Input: dimensioned drawing with shaded views. Units: mm. Origin: part minimum x, y, z. Round coordinates to 2 decimals unless told otherwise and drop trailing zeros. Loops run counter-clockwise (first coordinate to the right, second up) from the corner with the lowest first, then second, coordinate; pieces in that order, holes last.
Item 1: First-contact query: P1, Ø1.4, axis at y = 161.5, z = 1, coming from the +X side. Flat tip, straight axial feed; report the tip coordinate or a pass-through.
Item 2: Section query A-A on z = 2.25. Return loops of the section in (x, y) (1 decimal), then the cut area to 3 significant figures.
Item 3: Ray query, L1, parallel to Y at x = 16.75, z = 2.95 (1 decimal); L2, parallel to X at y = 33, z = 0.9. Return the intervals inside material, ascending.
Item 4: Section query B-B on y = 147. Return loops of the section in (x, z).
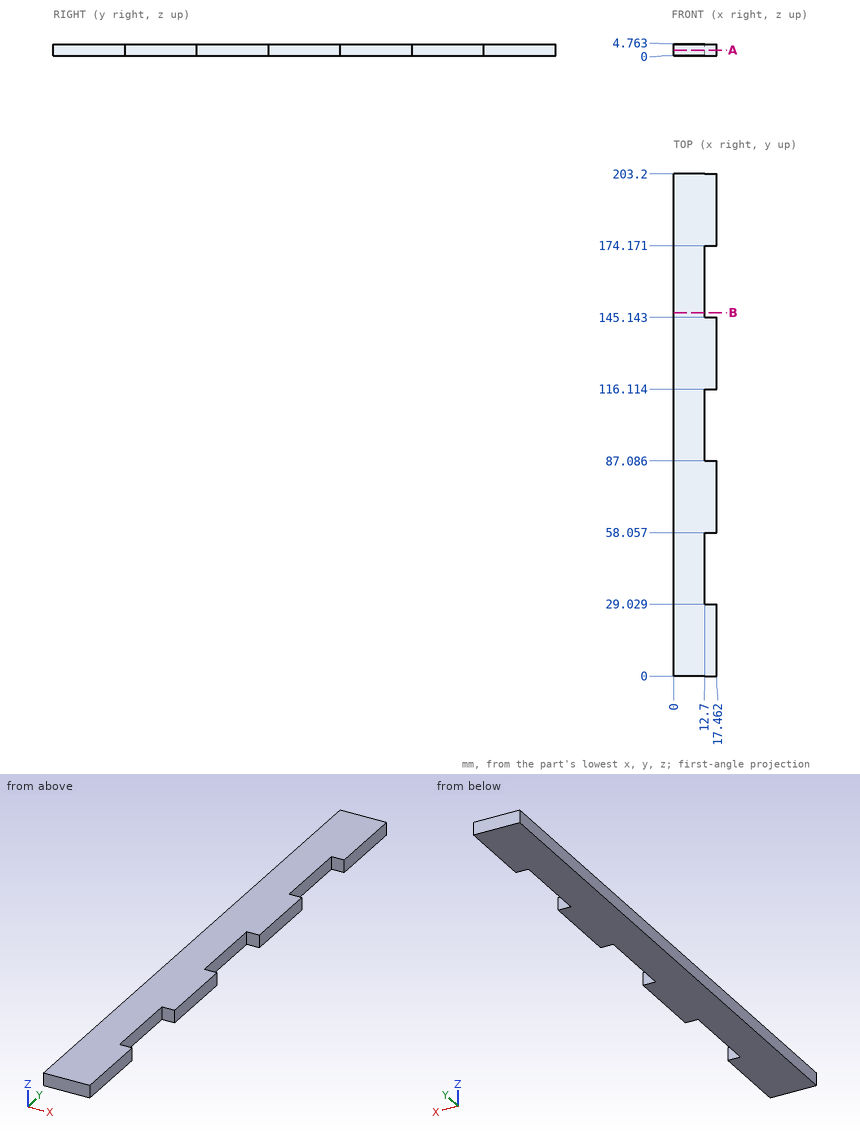
Data:
1. P1: stops at x = 12.7
2. outline: (0, 0) - (17.5, 0) - (17.5, 29) - (12.7, 29) - (12.7, 58.1) - (17.5, 58.1) - (17.5, 87.1) - (12.7, 87.1) - (12.7, 116.1) - (17.5, 116.1) - (17.5, 145.1) - (12.7, 145.1) - (12.7, 174.2) - (17.5, 174.2) - (17.5, 203.2) - (0, 203.2) - close
2. area: 3,130 mm2
3. L1: y = 0 to 29, 58.1 to 87.1, 116.1 to 145.1, 174.2 to 203.2
3. L2: x = 0 to 12.7
4. outline: (0, 0) - (12.7, 0) - (12.7, 4.76) - (0, 4.76) - close
